```python
from build123d import *

# Parameters (mm, degrees)
SKIZZE1_W                       = 37
SKIZZE1_H                       = 26.5
AUFSATZ_LINEAR_AUSTRAGEN1_DEPTH = 18
SKIZZE5_W                       = 33
SKIZZE5_H                       = 14
SCHNITT_LINEAR_AUSTRAGEN1_DEPTH = 28
SKIZZE6_R                       = 1.5
SCHNITT_LINEAR_AUSTRAGEN2_DEPTH = 4


with BuildPart() as part:
    # Skizze1 → Aufsatz-Linear austragen1 (new body)
    with BuildSketch(Plane(origin=(0, 0, 0), x_dir=(1, 0, 0), z_dir=(0, 1, 0))):
        Rectangle(SKIZZE1_W, SKIZZE1_H)
    extrude(amount=AUFSATZ_LINEAR_AUSTRAGEN1_DEPTH)

    # Skizze5 → Schnitt-Linear austragen1 (cut)
    with BuildSketch(Plane(origin=(0, 0, -11.25), x_dir=(-1, 0, 0), z_dir=(0, 0, -1))):
        with Locations((0, 9)):
            Rectangle(SKIZZE5_W, SKIZZE5_H)
    extrude(amount=-SCHNITT_LINEAR_AUSTRAGEN1_DEPTH, mode=Mode.SUBTRACT)

    # Skizze6 → Schnitt-Linear austragen2 (cut, symmetric)
    with BuildSketch(Plane.XZ):
        with Locations((-7, 8.75)):
            Circle(SKIZZE6_R)
        with Locations((7, 8.75)):
            Circle(SKIZZE6_R)
        with Locations((0, 8.75)):
            Circle(SKIZZE6_R)
    schnitt_linear_austragen2 = extrude(amount=SCHNITT_LINEAR_AUSTRAGEN2_DEPTH, both=True, mode=Mode.SUBTRACT)

    # Spiegeln1: Schnitt-Linear austragen2 across plane
    add(schnitt_linear_austragen2.mirror(Plane.XY), mode=Mode.SUBTRACT)


solid = part.part
```
Geometry check sheet. Reference: the model listing, model coordinates, mm. A direction names the side the tool comes from. Coordinates: 2 decimals unless noted, no trailing zeros. Order: outer loops, then holes, each group sorted by start corner. A loop starts at its lowest first (then second) coordinate and runs counter-clockwise, first axis right, second up. Notation, with made-up numbers: (69, 88) - (127, 88) arc R26 ccw to (127, 117) - close; hole circle Ø4 at (21, 50.5). An arc over 180 degrees is marked (long way). Answer as a JSON object with one key per item and string values. Group by question number.
Item 1: Sectioned sample at C-C, the plane y = 9.5. Record the cut outline in (x, z).
Item 2: Sectioned sample at D-D, the plane z = 1.5. Record the cut outline in (x, y), and give its area (3 significant figures).
Item 3: Sectioned sample at A-A, the plane z = 8.75. Record the cut outline in (x, y), and give its area (3 significant figures).
Item 4: Draft check along Y on faces 4 (the face through (0, 9, -13.25)), 5 (the face through (0, 18, 0)), 6 (the face through (0, 16, 1)), 7 (the face through (0, 9, -11.25)). Enter one of: +Y half, -Y half, draft (parallel to the pull), parting line (faces both ways), or undercut.
Item 5: Sectioned sample at B-B, the plane x = 0. Record the cut outline in (y, z).
Item 6: Scan lines: probe 1 along Z at (x, y) = (7, 0.65); probe 2 along Y at (x, z) = (-3.5, 4); probe 3 along X at (y, z) = (13.5, 1). Record each from-to range of solid material in increasing order.
Item 7: Depth check by flat-ended pin: pin 1 Ø2.5 at (x, z) = (7, 8.75) entering from -Y. Enter the tip coordinate at first touch or a pass-through.
Item 8: Tool access check on faces 1 (the face through (5.81, 0.99, -7.84)), 2 (the face through (0, 2, 1)), 3 (the face through (0, 0, 0)). Record the directions out of +Z, -Z, +X, -X, +Y, -Y that give a thin tool (end or side, any length) a straight path to the whole face; none if there is none.
Resolved:
{
 "1": {"outline": "(-18.5, -13.25) - (18.5, -13.25) - (18.5, 13.25) - (16.5, 13.25) - (16.5, -11.25) - (-16.5, -11.25) - (-16.5, 13.25) - (-18.5, 13.25) - close"},
 "2": {"outline": "(-18.5, 0) - (18.5, 0) - (18.5, 18) - (-18.5, 18) - close; hole (-16.5, 2) - (16.5, 2) - (16.5, 16) - (-16.5, 16) - close", "area": "204 mm^2"},
 "3": {"outline": "(-18.5, 0) - (-8.5, 0) - (-8.5, 2) - (-16.5, 2) - (-16.5, 16) - (16.5, 16) - (16.5, 2) - (8.5, 2) - (8.5, 0) - (18.5, 0) - (18.5, 18) - (-18.5, 18) - close; (-5.5, 0) - (-1.5, 0) - (-1.5, 2) - (-5.5, 2) - close; (1.5, 0) - (5.5, 0) - (5.5, 2) - (1.5, 2) - close", "area": "186 mm^2"},
 "4": {"face 4": "draft", "face 5": "+Y half", "face 6": "undercut", "face 7": "undercut"},
 "5": {"outline": "(0, -13.25) - (18, -13.25) - (18, 13.25) - (16, 13.25) - (16, -11.25) - (2, -11.25) - (2, -10.25) - (0, -10.25) - close; (0, -7.25) - (2, -7.25) - (2, 7.25) - (0, 7.25) - close; (0, 10.25) - (2, 10.25) - (2, 13.25) - (0, 13.25) - close"},
 "6": {"probe 1": "-13.25 to -10.25, -7.25 to 7.25, 10.25 to 13.25", "probe 2": "0 to 2, 16 to 18", "probe 3": "-18.5 to -16.5, 16.5 to 18.5"},
 "7": {"pin 1": "y = 16"},
 "8": {"face 1": "-Y", "face 2": "+Z", "face 3": "+Z, -Z, +X, -X, -Y"}
}
